Geometry check sheet. Reference: the model listing, model coordinates, mm. A direction names the side the tool comes from. Give positions to 0.01 mm unless a question says otherwise; leave off trailing zeros. Loops run counter-clockwise (first coordinate to the right, second up) from the corner with the lowest first, then second, coordinate; pieces in that order, holes last. Notation, with made-up numbers: (9.5, -35) - (35.5, -35) arc R23 ccw to (35.5, -11) - close; hole circle Ø10 at (-33.5, -40). An arc over 180 degrees is marked (long way). Use a Markdown table: item, result. Add a question column.
1. Cross-section at A-A on y = -16. Enter the section's corners in (x, z), and give its area (3 significant figures).
2. Cross-section at C-C on y = -66. Enter the section's corners in (x, z), and give its area (3 significant figures).
3. Set-up check for faces 5 (the cylindrical face through (40.4, -5.7, 1)), 6 (the cylindrical face through (65.575, -23.507, 17.553)), 7 (the flat face through (17, -191, 17)): record each of +Z, -Z, +X, -X, +Y, -Y from which the full face is reachable in a straight line by a thin tool's end or side.
4. Material ranges on L1, parallel to Y at x = 5.5, z = 25; L2, parallel to Y at x = -34, z = 7.5; L3, parallel to X at y = -28.5, z = 7, recorded low to high.
5. Depth check by flat-ended pin: P1, Ø6.5, axis at x = -58.14, y = -110, coming from the +Z side; P2, Ø2, axis at x = -2.5, z = 0.5, coming from the -Y side; P3, Ø2, axis at x = -31, z = 19.5, coming from the +Y side. Enter the tip coordinate at first touch or a pass-through.
6. Draft check along X on faces 1 (the flat face through (8, -27, 32)), 2 (the cylindrical face through (30.274, -58.017, 0.986)), 3 (the flat face through (-62.138, -27, 17)), 4 (the flat face through (80.862, -189, 17)). Enter one of: pulls with the +X half, pulls with the -X half, needs draft (parallel to the pull), parting line crosses it, or undercut.
from build123d import *

# Parameters (mm, degrees)
SZKIC4_R                    = 2
DODANIE_WYCI_GNI_CIE1_DEPTH = 2
DODANIE_WYCI_GNI_CIE2_DEPTH = 30
SZKIC6_W                    = 35
SZKIC6_H                    = 10
DODANIE_WYCI_GNI_CIE3_DEPTH = 2
SZKIC7_R                    = 11
WYTNIJ_WYCI_GNI_CIE1_DEPTH  = 7
SZKIC7_4_R                  = 11
WYTNIJ_WYCI_GNI_CIE2_DEPTH  = 7
SZKIC7_5_R                  = 11
WYTNIJ_WYCI_GNI_CIE3_DEPTH  = 7
SZKIC12_W                   = 145
SZKIC12_H                   = 8
DODANIE_WYCI_GNI_CIE5_DEPTH = 30
SZKIC13_R                   = 4.25
WYTNIJ_WYCI_GNI_CIE9_DEPTH  = 59
WYTNIJ_WYCI_GNI_CIE10_START = -7
SZKIC13_3_R                 = 11
WYTNIJ_WYCI_GNI_CIE10_DEPTH = 7
WYTNIJ_WYCI_GNI_CIE11_DEPTH = 178


with BuildPart() as part:
    # Szkic4 → Dodanie-wyciągnięcie1 (new body)
    with BuildSketch(Plane.XY):
        Polygon((71.861585453, -220), (81.861585453, -220), (81.861585453, 0), (-63.138414547, 0), (-63.138414547, -220), (-53.138414547, -220), (-53.138414547, -31), (-18.138414547, -31), (-18.138414547, -220), (-8.138414547, -220), (-8.138414547, -31), (26.861585453, -31), (26.861585453, -220), (36.861585453, -220), (36.861585453, -31), (71.861585453, -31), align=None)
        with Locations((76.861585453, -3.6)):
            Circle(SZKIC4_R, mode=Mode.SUBTRACT)
        with Locations((31.861585453, -3.6)):
            Circle(SZKIC4_R, mode=Mode.SUBTRACT)
        with Locations((-13.138414547, -3.6)):
            Circle(SZKIC4_R, mode=Mode.SUBTRACT)
        with Locations((-58.138414547, -3.6)):
            Circle(SZKIC4_R, mode=Mode.SUBTRACT)
        with Locations((76.861585453, -56.8)):
            Circle(SZKIC4_R, mode=Mode.SUBTRACT)
        with Locations((31.861585453, -56.8)):
            Circle(SZKIC4_R, mode=Mode.SUBTRACT)
        with Locations((-13.138414547, -56.8)):
            Circle(SZKIC4_R, mode=Mode.SUBTRACT)
        with Locations((76.861585453, -110)):
            Circle(SZKIC4_R, mode=Mode.SUBTRACT)
        with Locations((31.861585453, -110)):
            Circle(SZKIC4_R, mode=Mode.SUBTRACT)
        with Locations((-13.138414547, -110)):
            Circle(SZKIC4_R, mode=Mode.SUBTRACT)
        with Locations((76.861585453, -163.2)):
            Circle(SZKIC4_R, mode=Mode.SUBTRACT)
        with Locations((31.861585453, -163.2)):
            Circle(SZKIC4_R, mode=Mode.SUBTRACT)
        with Locations((-13.138414547, -163.2)):
            Circle(SZKIC4_R, mode=Mode.SUBTRACT)
        with Locations((76.861585453, -216.4)):
            Circle(SZKIC4_R, mode=Mode.SUBTRACT)
        with Locations((31.861585453, -216.4)):
            Circle(SZKIC4_R, mode=Mode.SUBTRACT)
        with Locations((-13.138414547, -216.4)):
            Circle(SZKIC4_R, mode=Mode.SUBTRACT)
        with Locations((-58.138414547, -56.8)):
            Circle(SZKIC4_R, mode=Mode.SUBTRACT)
        with Locations((-58.138414547, -110)):
            Circle(SZKIC4_R, mode=Mode.SUBTRACT)
        with Locations((-58.138414547, -163.2)):
            Circle(SZKIC4_R, mode=Mode.SUBTRACT)
        with Locations((-58.138414547, -216.4)):
            Circle(SZKIC4_R, mode=Mode.SUBTRACT)
        with BuildLine():
            Line((-48.238414547, -12), (-48.238414547, -10.049358869))
            ThreePointArc((-48.238414547, -10.049358869), (-49.638414547, -5.7), (-51.038414547, -10.049358869))
            Line((-51.038414547, -10.049358869), (-51.038414547, -12))
            Line((-51.038414547, -12), (-53.138414547, -12))
            Line((-53.138414547, -12), (-53.138414547, -23))
            Line((-53.138414547, -23), (-46.138414547, -23))
            Line((-46.138414547, -23), (-46.138414547, -12))
            Line((-46.138414547, -12), (-48.238414547, -12))
        make_face(mode=Mode.SUBTRACT)
        with BuildLine():
            Line((-3.238414547, -12), (-3.238414547, -10.049358869))
            ThreePointArc((-3.238414547, -10.049358869), (-4.638414547, -5.7), (-6.038414547, -10.049358869))
            Line((-6.038414547, -10.049358869), (-6.038414547, -12))
            Line((-6.038414547, -12), (-8.138414547, -12))
            Line((-8.138414547, -12), (-8.138414547, -23))
            Line((-8.138414547, -23), (-1.138414547, -23))
            Line((-1.138414547, -23), (-1.138414547, -12))
            Line((-1.138414547, -12), (-3.238414547, -12))
        make_face(mode=Mode.SUBTRACT)
        with BuildLine():
            Line((41.761585453, -12), (41.761585453, -10.049358869))
            ThreePointArc((41.761585453, -10.049358869), (40.361585453, -5.7), (38.961585453, -10.049358869))
            Line((38.961585453, -10.049358869), (38.961585453, -12))
            Line((38.961585453, -12), (36.861585453, -12))
            Line((36.861585453, -12), (36.861585453, -23))
            Line((36.861585453, -23), (43.861585453, -23))
            Line((43.861585453, -23), (43.861585453, -12))
            Line((43.861585453, -12), (41.761585453, -12))
        make_face(mode=Mode.SUBTRACT)
    extrude(amount=DODANIE_WYCI_GNI_CIE1_DEPTH)

    # Szkic5 → Dodanie-wyciągnięcie2 (add)
    with BuildSketch(Plane.XY.offset(2)):
        Polygon((-63.138414547, -192), (-63.138414547, -194), (81.861585453, -194), (81.861585453, -184), (-63.138414547, -184), (-63.138414547, -185), align=None)
    extrude(amount=DODANIE_WYCI_GNI_CIE2_DEPTH)

    # Szkic6 → Dodanie-wyciągnięcie3 (add)
    with BuildSketch(Plane(origin=(0, 0, 2), x_dir=(-1, 0, 0), z_dir=(0, 0, -1))):
        with Locations((35.638414547, -189)):
            Rectangle(SZKIC6_W, SZKIC6_H)
        with Locations((-9.361585453, -189)):
            Rectangle(SZKIC6_W, SZKIC6_H)
        with Locations((-54.361585453, -189)):
            Rectangle(SZKIC6_W, SZKIC6_H)
    extrude(amount=DODANIE_WYCI_GNI_CIE3_DEPTH)

    # Szkic7 → Wytnij-wyciągnięcie1 (cut)
    with BuildSketch(Plane(origin=(0, -184, 0), x_dir=(1, 0, 0), z_dir=(0, 1, 0))):
        with Locations(Location((61.361585453, -17, 0), (0, 0, 270))):
            Circle(SZKIC7_R)
    extrude(amount=-WYTNIJ_WYCI_GNI_CIE1_DEPTH, mode=Mode.SUBTRACT)

    # Szkic7<4> → Wytnij-wyciągnięcie2 (cut)
    with BuildSketch(Plane(origin=(0, -184, 0), x_dir=(1, 0, 0), z_dir=(0, 1, 0))):
        with Locations(Location((16.361585453, -17, 0), (0, 0, 270))):
            Circle(SZKIC7_4_R)
    extrude(amount=-WYTNIJ_WYCI_GNI_CIE2_DEPTH, mode=Mode.SUBTRACT)

    # Szkic7<5> → Wytnij-wyciągnięcie3 (cut)
    with BuildSketch(Plane(origin=(0, -184, 0), x_dir=(1, 0, 0), z_dir=(0, 1, 0))):
        with Locations(Location((-28.638414547, -17, 0), (0, 0, 270))):
            Circle(SZKIC7_5_R)
    extrude(amount=-WYTNIJ_WYCI_GNI_CIE3_DEPTH, mode=Mode.SUBTRACT)

    # Szkic12 → Dodanie-wyciągnięcie5 (add)
    with BuildSketch(Plane.XY.offset(2)):
        with Locations((9.361585453, -27)):
            Rectangle(SZKIC12_W, SZKIC12_H)
    extrude(amount=DODANIE_WYCI_GNI_CIE5_DEPTH)

    # Szkic13 → Wytnij-wyciągnięcie9 (cut)
    with BuildSketch(Plane.XZ.offset(31)):
        with Locations(Location((61.361585453, 17, 0), (0, 0, 270))):
            Circle(SZKIC13_R)
        with Locations(Location((16.361585453, 17, 0), (0, 0, 270))):
            Circle(SZKIC13_R)
        with Locations(Location((-28.638414547, 17, 0), (0, 0, 270))):
            Circle(SZKIC13_R)
    extrude(amount=-WYTNIJ_WYCI_GNI_CIE9_DEPTH, mode=Mode.SUBTRACT)

    # Szkic13<3> → Wytnij-wyciągnięcie10 (cut)
    with BuildSketch(Plane.XZ.offset(31).offset(WYTNIJ_WYCI_GNI_CIE10_START)):
        with Locations(Location((61.361585453, 17, 0), (0, 0, 90))):
            Circle(SZKIC13_3_R)
        with Locations(Location((16.361585453, 17, 0), (0, 0, 90))):
            Circle(SZKIC13_3_R)
        with Locations(Location((-28.638414547, 17, 0), (0, 0, 90))):
            Circle(SZKIC13_3_R)
    extrude(amount=WYTNIJ_WYCI_GNI_CIE10_DEPTH, mode=Mode.SUBTRACT)

    # Szkic14 → Wytnij-wyciągnięcie11 (cut)
    with BuildSketch(Plane.XZ.offset(194)):
        Polygon((-63.138414547, 2), (-62.138414547, 2), (-62.138414547, 31), (-62.138414547, 32), (-63.138414547, 32), align=None)
        Polygon((80.861585453, 31), (80.861585453, 2), (81.861585453, 2), (81.861585453, 32), (80.861585453, 32), align=None)
    extrude(amount=-WYTNIJ_WYCI_GNI_CIE11_DEPTH, mode=Mode.SUBTRACT)


solid = part.part
Values found:
| question | item | result |
|---|---|---|
| 1 | outline | (-63.14, 0) - (-53.14, 0) - (-53.14, 2) - (-63.14, 2) - close; (-46.14, 0) - (-8.14, 0) - (-8.14, 2) - (-46.14, 2) - close; (-1.14, 0) - (36.86, 0) - (36.86, 2) - (-1.14, 2) - close; (43.86, 0) - (81.86, 0) - (81.86, 2) - (43.86, 2) - close |
| 1 | area | 248 mm2 |
| 2 | outline | (-63.14, 0) - (-53.14, 0) - (-53.14, 2) - (-63.14, 2) - close; (-18.14, 0) - (-8.14, 0) - (-8.14, 2) - (-18.14, 2) - close; (26.86, 0) - (36.86, 0) - (36.86, 2) - (26.86, 2) - close; (71.86, 0) - (81.86, 0) - (81.86, 2) - (71.86, 2) - close |
| 2 | area | 80.0 mm2 |
| 3 | face 5 | +Z, -Z |
| 3 | face 6 | +Y |
| 3 | face 7 | none |
| 4 | L1 | y = -194 to -184, -31 to -23 |
| 4 | L2 | y = -194 to -191, -24 to -23 |
| 4 | L3 | x = -62.14 to -33.22, -24.06 to 11.78, 20.94 to 56.78, 65.94 to 80.86 |
| 5 | P1 | stops at z = 2 |
| 5 | P2 | stops at y = -194 |
| 5 | P3 | stops at y = -23 |
| 6 | face 1 | needs draft |
| 6 | face 2 | undercut |
| 6 | face 3 | pulls with the -X half |
| 6 | face 4 | pulls with the +X half |
